Geometry: see drawing. Coordinates: mm, zero at the bounding-box minimum. Coordinates: 2 decimals unless noted, no trailing zeros. Loops run counter-clockwise (first coordinate to the right, second up) from the corner with the lowest first, then second, coordinate; pieces in that order, holes last. Notation, with made-up numbers: (-15.75, -4) - (37.25, -4) arc R27 cw to (37.25, 16) - close; hole circle Ø9 at (26.5, 66). An arc over 180 degrees is marked (long way). Answer in a Markdown table with one row per item.
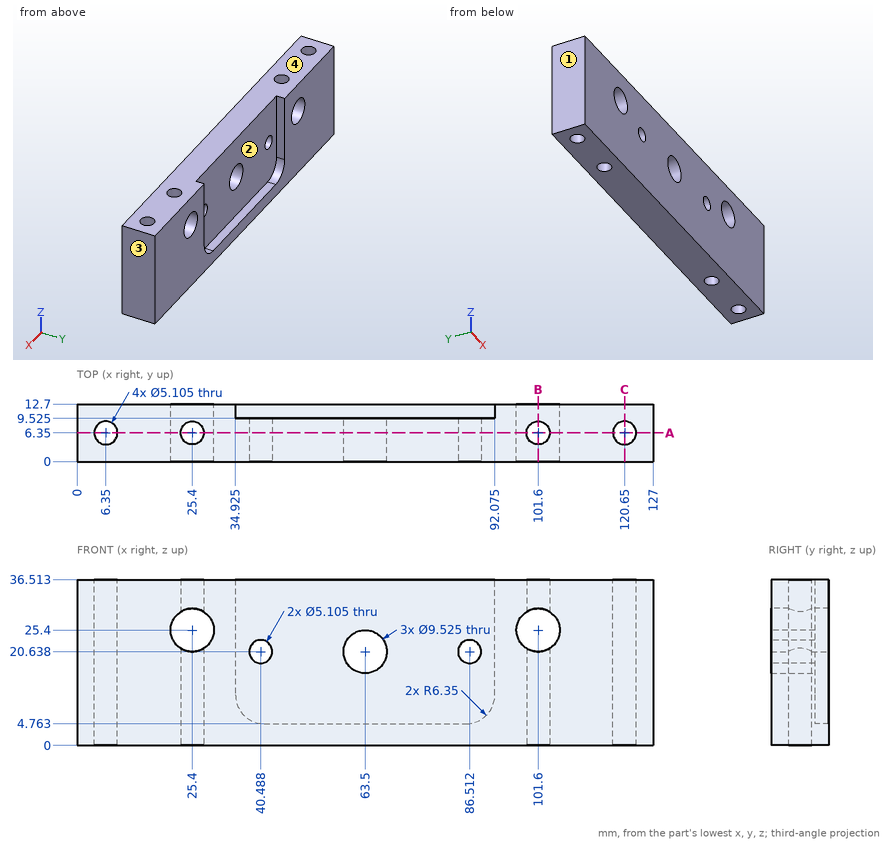
(1) Cut plane C-C on x = 120.65. Output: boundary loops of the cut face in (y, z).
Verdict:
| item | result |
|---|---|
| outline | (0, 0) - (3.8, 0) - (3.8, 36.51) - (0, 36.51) - close; (8.9, 0) - (12.7, 0) - (12.7, 36.51) - (8.9, 36.51) - close |
(2) Ray query, probe 1 along X at (y, z) = (7, 8); probe 2 along X at (y, z) = (10.25, 28) (1 decimal); probe 3 along Z at (x, y) = (63, 9.25). Return the intervals inside material, ascending.
Verdict:
| item | result |
|---|---|
| probe 1 | x = 0 to 3.88, 8.82 to 22.93, 27.87 to 99.13, 104.07 to 118.18, 123.12 to 127 |
| probe 2 | x = 0 to 21.4, 29.4 to 34.9, 92.1 to 97.6, 105.6 to 127 |
| probe 3 | z = 0 to 15.9, 25.37 to 36.51 |
(3) First-contact query: pin 1 Ø15 at (x, z) = (63.5, 20.64) entering from +Y (1 decimal); pin 2 Ø11 at (x, z) = (101.6, 25.4) entering from -Y; pin 3 Ø2.5 at (x, y) = (66.5, 11.5) entering from +Z. Flat tips, straight axial feed; report the tip coordinate or a pass-through.
Verdict:
| item | result |
|---|---|
| pin 1 | stops at y = 9.5 |
| pin 2 | stops at y = 0 |
| pin 3 | stops at z = 4.76 |
(4) Cut plane B-B on x = 101.6. Output: boundary loops of the cut face in (y, z), then the cut area to 3 significant figures.
Verdict:
| item | result |
|---|---|
| outline | (0, 0) - (3.8, 0) - (3.8, 20.64) - (0, 20.64) - close; (0, 30.16) - (3.8, 30.16) - (3.8, 36.51) - (0, 36.51) - close; (8.9, 0) - (12.7, 0) - (12.7, 20.64) - (8.9, 20.64) - close; (8.9, 30.16) - (12.7, 30.16) - (12.7, 36.51) - (8.9, 36.51) - close |
| area | 205 mm² |
(5) Pull-direction query (X, two-part tool) for the marked faces 1, 2, 3 and 4; classes: pulls with the +X half, pulls with the -X half, needs draft (parallel to the pull), parting line crosses it, or undercut.
Verdict:
| item | result |
|---|---|
| face 1 | pulls with the -X half |
| face 2 | undercut |
| face 3 | pulls with the +X half |
| face 4 | needs draft |
(6) Cut plane A-A on y = 6.35. State how many separate pieces and enclosed holes the cut face has, then the cut area to 3 significant figures.
Verdict:
| item | result |
|---|---|
| separate pieces | 5 |
| enclosed holes | 3 |
| area | 3,730 mm² |
